Model file for the job. Use its own axes, mm. A direction names the side the tool comes from. Round coordinates to 2 decimals unless told otherwise and drop trailing zeros. Loops run counter-clockwise (first coordinate to the right, second up) from the corner with the lowest first, then second, coordinate; pieces in that order, holes last. Notation, with made-up numbers: (15, 39) - (67, 39) arc R12 cw to (67, 51) - close; hole circle Ø4 at (0, -8.75). An arc over 180 degrees is marked (long way). Answer as a JSON object with one key per item and string values.
from build123d import *

# Parameters (mm, degrees)
SKETCH1_W           = 70
SKETCH1_H           = 42.5
BOSS_EXTRUDE1_DEPTH = 2
BOSS_EXTRUDE2_DEPTH = 21
SKETCH3_W           = 2
SKETCH3_H           = 12.5
BOSS_EXTRUDE3_DEPTH = 11
FILLET2_R           = 1


with BuildPart() as part:
    # Sketch1 → Boss-Extrude1 (new body)
    with BuildSketch(Plane(origin=(0, 0, 0), x_dir=(1, 0, 0), z_dir=(0, 1, 0))):
        Rectangle(SKETCH1_W, SKETCH1_H)
    extrude(amount=-BOSS_EXTRUDE1_DEPTH)

    # Sketch2 → Boss-Extrude2 (add)
    with BuildSketch(Plane(origin=(0, 0, 0), x_dir=(-1, 0, 0), z_dir=(0, 1, 0))):
        Polygon((-33, 19.25), (33, 19.25), (33, 11), (35, 11), (35, 21.25), (-35, 21.25), (-35, -21.25), (35, -21.25), (35, -1.5), (33, -1.5), (33, -19.25), (-33, -19.25), align=None)
    extrude(amount=BOSS_EXTRUDE2_DEPTH)

    # Sketch3 → Boss-Extrude3 (add)
    with BuildSketch(Plane(origin=(0, 21, 0), x_dir=(1, 0, 0), z_dir=(0, 1, 0))):
        with Locations((-34, -4.75)):
            Rectangle(SKETCH3_W, SKETCH3_H)
    extrude(amount=-BOSS_EXTRUDE3_DEPTH)

    # Fillet2
    fillet2_edges = [part.edges().sort_by_distance(p)[0] for p in [
        (35, -2, 0),
        (-35, 0, 4.75),
        (0, -2, -21.25),
        (-33, 0, -10.375),
        (0, 0, -19.25),
        (-33, 10.5, -19.25),
        (33, 21, 0),
        (33, 10.5, -19.25),
        (0, 21, 19.25),
        (33, 10.5, 19.25),
        (-33, 0, 15.125),
        (-33, 10.5, 19.25),
        (-34, 0, 11),
        (-33, 21, 0),
        (0, 21, -19.25),
        (-34, 0, -1.5),
        (0, 0, 19.25),
        (33, 0, 0),
        (-35, 5, 11),
        (-33, 5, 11),
        (-33, 5, -1.5),
        (-35, 5, -1.5),
        (-35, -2, 0),
        (-33, 10, 4.75),
        (-35, 10, 4.75),
        (-35, 9.5, -21.25),
        (35, 9.5, -21.25),
        (35, 9.5, 21.25),
        (-35, 9.5, 21.25),
        (0, -2, 21.25),
    ]]
    fillet(fillet2_edges, radius=FILLET2_R - 0.0001)  # a hair under: the kernel refuses the full size


solid = part.part
1) Slice it at C-C on x = 4. List the corners of the cut face in (y, z).
Values follow:
{"outline": "(-2, -20.25) arc R1 ccw to (-1, -21.25) - (21, -21.25) - (21, -20.25) arc R1 ccw to (20, -19.25) - (1, -19.25) arc R1 cw to (0, -18.25) - (0, 18.25) arc R1 cw to (1, 19.25) - (20, 19.25) arc R1 ccw to (21, 20.25) - (21, 21.25) - (-1, 21.25) arc R1 ccw to (-2, 20.25) - close"}
2) Probe probe 1 along Z at (x, y) = (19, 2); probe 2 along X at (y, z) = (17.5, -8); probe 3 along Y at (x, z) = (-10, -9). List the from-to ranges inside material, lowest first.
Values follow:
{"probe 1": "-21.25 to -19.25, 19.25 to 21.25", "probe 2": "-35 to -33, 33 to 35", "probe 3": "-2 to 0"}
3) Tool access for faces 1 (the flat face through (0, 21, -21)), 2 (the flat face through (33, 10, 0)): list every direction of +Z, -Z, +X, -X, +Y, -Y with a clear straight run to the whole face (end or side of a thin tool).
Values follow:
{"face 1": "+Z, -Z, +X, -X, +Y", "face 2": "+Y"}
4) Slice it at B-B on y = 14. List the corners of the cut face in (x, z), then the cut area to 3 significant figures.
Values follow:
{"outline": "(-35, -20.25) arc R1 ccw to (-34, -21.25) - (34, -21.25) arc R1 ccw to (35, -20.25) - (35, 20.25) arc R1 ccw to (34, 21.25) - (-34, 21.25) arc R1 ccw to (-35, 20.25) - close; hole (-33, -18.25) arc R1 ccw to (-32, -19.25) - (32, -19.25) arc R1 ccw to (33, -18.25) - (33, 18.25) arc R1 ccw to (32, 19.25) - (-32, 19.25) arc R1 ccw to (-33, 18.25) - close", "area": "434 mm²"}
5) Two-plate mould, pull along Z, no slides. Class faces 3 (the flat face through (0, 10, 21.25)), 4 (the flat face through (35, 10, 0)), 5 (the flat face through (-33, 13, 0)), 6 (the flat face through (0, 10, -21.25)): pulls with the +Z half, pulls with the -Z half, needs draft (parallel to the pull), parting line crosses it, or undercut.
Values follow:
{"face 3": "pulls with the +Z half", "face 4": "needs draft", "face 5": "undercut", "face 6": "pulls with the -Z half"}
